from build123d import *

# Parameters (mm, degrees)
ESQUISSE1_W             = 15
ESQUISSE1_H             = 90
BOSS_EXTRU_1_DEPTH      = 10
ESQUISSE2_R             = 3
ESQUISSE2_R_2           = 2.6
ENL_V_MAT_EXTRU_1_DEPTH = 10
CONG_1_R                = 7.5
ENL_V_MAT_EXTRU_2_DEPTH = 92.787798753
ESQUISSE4_R             = 2.1
ENL_V_MAT_EXTRU_3_DEPTH = 92.787798753
ESQUISSE5_R             = 3
ENL_V_MAT_EXTRU_4_DEPTH = 6.5
CONG_2_R                = 1


with BuildPart() as part:
    # Esquisse1 → Boss.-Extru.1 (new body)
    with BuildSketch(Plane.XY):
        with Locations((7.5, 45)):
            Rectangle(ESQUISSE1_W, ESQUISSE1_H)
    extrude(amount=BOSS_EXTRU_1_DEPTH)

    # Esquisse2 → Enlèv. mat.-Extru.1 (cut)
    with BuildSketch(Plane.XY.offset(10)):
        with Locations((7.5, 82)):
            Circle(ESQUISSE2_R)
        with Locations((7.5, 8)):
            Circle(ESQUISSE2_R_2)
    extrude(amount=-ENL_V_MAT_EXTRU_1_DEPTH, mode=Mode.SUBTRACT)

    # Congé1
    cong_1_edges = [part.edges().sort_by_distance(p)[0] for p in [
        (15, 90, 5),
        (0, 90, 5),
        (15, 0, 5),
        (0, 0, 5),
    ]]
    fillet(cong_1_edges, radius=CONG_1_R - 0.0001)  # a hair under: the kernel refuses the full size

    # Esquisse3 → Enlèv. mat.-Extru.2 (cut, through all)
    with BuildSketch(Plane.XY.offset(10)):
        Polygon((6.5, 10.4), (6.5, 31.228427125), (15, 39.728427125), (15, 36.9), (8.5, 30.4), (8.5, 10.4), align=None)
    extrude(amount=-ENL_V_MAT_EXTRU_2_DEPTH, mode=Mode.SUBTRACT)

    # Esquisse4 → Enlèv. mat.-Extru.3 (cut, through all)
    with BuildSketch(Plane(origin=(15, 0, 0), x_dir=(0, 0, -1), z_dir=(1, 0, 0))):
        with Locations((-5, 15.5)):
            Circle(ESQUISSE4_R)
        with Locations((-5, 25.5)):
            Circle(ESQUISSE4_R)
    extrude(amount=-ENL_V_MAT_EXTRU_3_DEPTH, mode=Mode.SUBTRACT)

    # Esquisse5 → Enlèv. mat.-Extru.4 (cut)
    with BuildSketch(Plane(origin=(15, 0, 0), x_dir=(0, 0, -1), z_dir=(1, 0, 0))):
        with Locations((-5, 25.5)):
            Circle(ESQUISSE5_R)
        with Locations((-5, 15.5)):
            Circle(ESQUISSE5_R)
    extrude(amount=-ENL_V_MAT_EXTRU_4_DEPTH, mode=Mode.SUBTRACT)

    # Congé2
    cong_2_edges = [part.edges().sort_by_distance(p)[0] for p in [
        (8.5, 10.4, 5),
        (6.5, 10.4, 5),
        (6.5, 31.228427125, 5),
        (15, 39.728427125, 5),
        (15, 36.9, 5),
        (8.5, 30.4, 5),
    ]]
    fillet(cong_2_edges, radius=CONG_2_R)


solid = part.part
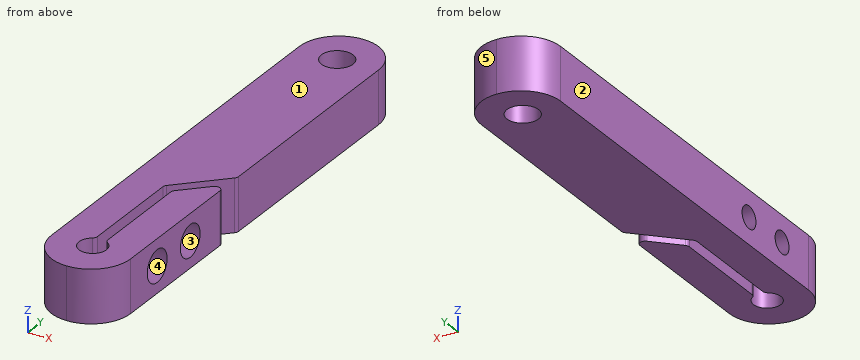
Model file for the job. Use its own axes, mm. Face numbers are marked on the shaded views. A direction names the side the tool comes from. Give positions to 0.01 mm unless a question says otherwise; leave off trailing zeros. Order: outer loops, then holes, each group sorted by start corner. A loop starts at its lowest first (then second) coordinate and runs counter-clockwise, first axis right, second up. Notation, with made-up numbers: (-38, 5) - (-30, 5) arc R22 cw to (-30, 34) - close; hole circle Ø5 at (18, 67.5). An arc over 180 degrees is marked (long way). Return JSON: item names as keys, results as strings.
1) Cut at C-C, the plane x = 3.5. Give the cut face in (y, z).
Geometry says:
{"outline": "(1.16, 0) - (88.84, 0) - (88.84, 10) - (1.16, 10) - close; hole circle Ø4.2 at (15.5, 5); hole circle Ø4.2 at (25.5, 5)"}
2) Probe line 1 (X direction, y = 12, z = 7.25); line 2 (X direction, y = 8, z = 2); line 3 (Y direction, x = 7.5, z = 6.75). List the from-to ranges inside material, lowest first. Write a range as from..to.
Geometry says:
{"line 1": "0..6.5, 8.5..15", "line 2": "0..4.9, 10.1..15", "line 3": "0..5.4, 32.23..79, 85..90"}
3) Pull direction Z, two halves, no side cores. Call the marked faces 1, 2 and 3: pulls with the +Z half, pulls with the -Z half, needs draft (parallel to the pull), parting line crosses it, or undercut.
Geometry says:
{"face 1": "pulls with the +Z half", "face 2": "needs draft", "face 3": "undercut"}
4) Cut at B-B, the plane z = 5. Count the separate pieces of the cut face and the enclosed holes in it, plus the area to 3 significant figures.
Geometry says:
{"separate pieces": "5", "enclosed holes": "1", "area": "1,060 mm²"}
5) Cut at A-A, the plane y = 25.5. Give the cut face in (x, z).
Geometry says:
{"outline": "(0, 0) - (6.5, 0) - (6.5, 2.9) - (0, 2.9) - close; (0, 7.1) - (6.5, 7.1) - (6.5, 10) - (0, 10) - close; (8.5, 0) - (15, 0) - (15, 2) - (8.5, 2) - close; (8.5, 8) - (15, 8) - (15, 10) - (8.5, 10) - close"}
6) Flat gauge pins, fed straight in: P1, Ø3, axis at x = 5, z = 6, coming from the +Y side; P2, Ø1.5, axis at x = 13, z = 2, coming from the -Y side; P3, Ø5.5, axis at y = 15.5, z = 5, coming from the +X side. Where does each tip first touch, or does it go through?
Geometry says:
{"P1": "y = 89.93", "P2": "y = 1.7", "P3": "x = 6.5"}
7) 3-axis set-ups, long thin cutter, end or side, ignore diameter. For the marked faces 4 and 5: which of +Z, -Z, +X, -X, +Y, -Y reach the whole face in a straight line?
Geometry says:
{"face 4": "+X", "face 5": "+Z, -Z, +X, +Y"}
